The listing builds one solid part. Answer for the finished solid, in the listing's coordinates (mm). Face numbers are marked on the shaded views. A direction names the side the tool comes from. Round coordinates to 2 decimals unless told otherwise and drop trailing zeros. Loops run counter-clockwise (first coordinate to the right, second up) from the corner with the lowest first, then second, coordinate; pieces in that order, holes last. Notation, with made-up numbers: (-39.75, 49) -> (-7.75, 49) arc R25 ccw to (-7.75, 85) -> close; hole circle Ø7 at (53.25, 21.5). An arc over 180 degrees is marked (long way). Answer in a Markdown table with one row per item. Add a question column.
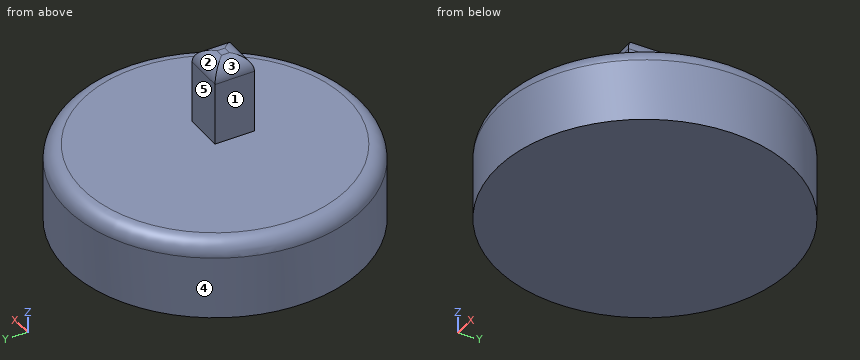
```python
from build123d import *

# Parameters (mm, degrees)
F0_R     = 47.934671
F1_DEPTH = 25.4
F2_W     = 12.7
F2_H     = 12.7
F3_DEPTH = 25.4
F4_R     = 5.08


with BuildPart() as f1:
    # F0 (on Top) → F1 (new body)
    with BuildSketch(Plane.XY):
        Circle(F0_R)
    extrude(amount=F1_DEPTH)

    # F2 (on face) → F3 (join)
    with BuildSketch(Plane.XY.offset(25.4)):
        with Locations((6.35, -6.35)):
            Rectangle(F2_W, F2_H)
    extrude(amount=F3_DEPTH)

    # F4
    f4_edges = [f1.edges().sort_by_distance(p)[0] for p in [
        (-47.934671, 0, 25.4),
        (6.35, -12.7, 50.8),
        (12.7, -6.35, 50.8),
        (6.35, 0, 50.8),
        (0, -6.35, 50.8),
    ]]
    fillet(f4_edges, radius=F4_R)


solid = f1.part
```
Item 1: The mould has two halves that part along X. Classify the marked faces 3, 4 and 5: +X half, -X half, draft (parallel to the pull), parting line (faces both ways), or undercut.
Item 2: For the marked faces 1 and 2, determine the directions among +Z, -Z, +X, -X, +Y, -Y from which every point of the face is accessible in a straight line to the end or side of a thin tool.
Item 3: Flat-ended cylindrical pins translate along their axes: P1, Ø10, axis at x = -8.5, z = 32, coming from the +Y side; P2, Ø1.5, axis at x = -15, y = 9.5, coming from the +Z side; P3, Ø2, axis at x = 4.5, z = 15.5, coming from the -Y side; P4, Ø14, axis at x = 8.5, z = 34, coming from the -Y side. Find the tip coordinate at first contact, or state that the pin passes through.
Item 4: Section B-B, the plane z = 23 is taken. Write down the section's boundary in (x, y).
Item 5: Section A-A, the plane z = 39 is taken. Write down the section's boundary in (x, y).
Item 6: Consider L1, parallel to Z at x = -37, y = -9.5; L2, parallel to Y at x = 7, z = 48.5; L3, parallel to Z at x = -10, y = 43.5. Determine where each line is inside the solid, lowest interval first. Write a range as from..to.
Here are the results:
| question | item | result |
|---|---|---|
| 1 | face 3 | -X half |
| 1 | face 4 | parting line |
| 1 | face 5 | draft |
| 2 | face 1 | +Z, -X, +Y, -Y |
| 2 | face 2 | +Z, +X, -X, +Y |
| 3 | P1 | passes through |
| 3 | P2 | stops at z = 25.4 |
| 3 | P3 | stops at y = -47.81 |
| 3 | P4 | stops at y = -12.7 |
| 4 | outline | circle Ø94.34 at (0, 0) |
| 5 | outline | (0, -12.7) -> (12.7, -12.7) -> (12.7, 0) -> (0, 0) -> close |
| 6 | L1 | z = 0..25.4 |
| 6 | L2 | y = -11.87..-0.83 |
| 6 | L3 | z = 0..25.08 |
